from build123d import *

# Parameters (mm, degrees)
SKETCH8_R           = 2.38125
SKETCH8_R_2         = 1.82245
SKETCH10_R          = 2.38125
BOSS_EXTRUDE3_DEPTH = 1.778
BOSS_EXTRUDE3_TAPER = -37
SKETCH11_R          = 1.82245
CUT_EXTRUDE2_DEPTH  = 2.7780001
CUT_EXTRUDE2_TAPER  = -37


with BuildPart() as part:
    # Sweep2: sweep along a path in Sketch9
    with BuildLine(Plane(origin=(0, 0, 0), x_dir=(0, 0, -1), z_dir=(1, 0, 0))) as sweep2_path:
        Line((-19.702223994, -95.902223994), (-19.702223994, -19.702223994))
        ThreePointArc((-19.702223994, -19.702223994), (-13.931576191, -5.770647803), (0, 0))
    # Sketch8 → Sweep2 (sweep)
    with BuildSketch(Plane.XY):
        Circle(SKETCH8_R)
        Circle(SKETCH8_R_2, mode=Mode.SUBTRACT)
    sweep2 = sweep(path=sweep2_path.line)

    # Sketch10 → Boss-Extrude3 (add)
    with BuildSketch(Plane.XZ.offset(95.902223994)):
        with Locations((0, 19.702223994)):
            Circle(SKETCH10_R)
    boss_extrude3 = extrude(amount=BOSS_EXTRUDE3_DEPTH, taper=BOSS_EXTRUDE3_TAPER)

    # Sketch11 → Cut-Extrude2 (cut, through all)
    with BuildSketch(Plane(origin=(0, -95.902223994, 0), x_dir=(1, 0, 0), z_dir=(0, 1, 0))):
        with Locations(Location((0, -19.702223994, 0), (0, 0, 270))):  # turned: the seam where the file's is
            Circle(SKETCH11_R)
    cut_extrude2 = extrude(amount=-CUT_EXTRUDE2_DEPTH, taper=CUT_EXTRUDE2_TAPER, mode=Mode.SUBTRACT)

    # Mirror1: Sweep2, Boss-Extrude3, Cut-Extrude2 across plane
    add(sweep2.mirror(Plane.XY))
    add(boss_extrude3.mirror(Plane.XY))
    add(cut_extrude2.mirror(Plane.XY), mode=Mode.SUBTRACT)


solid = part.part
Source: CAD feature listing. Evaluate the final solid. Frame: model axes, mm. A direction names the side the tool comes from. Round coordinates to 2 decimals unless told otherwise and drop trailing zeros. Loops run counter-clockwise (first coordinate to the right, second up) from the corner with the lowest first, then second, coordinate; pieces in that order, holes last. Notation, with made-up numbers: (-4.5, 45.25) - (23.5, 45.25) arc R36 cw to (23.5, 79.25) - close; hole circle Ø4 at (-29.75, -36). An arc over 180 degrees is marked (long way). Write item = value, one per line. Start each with the question number.
(1) Section query B-B, the plane y = -12.5. State how many separate pieces and enclosed holes the cut face has, plus the area to 3 significant figures.
(2) Ray query, line 1 along Z through (x, y) = (-0.25, -37.5); line 2 along X through (y, z) = (-33, 19.5); line 3 along Z through (x, y) = (-0.5, -71). Return the intervals inside material, ascending. Write a range as from..to.
(3) Pull-direction query (Z, two-part tool) for faces 3 (the face through (-0.237, -57.269, -17.895)), 4 (the face through (-0.237, -57.269, 17.895)), 5 (the face through (-2, -97.68, -17)); classes: +Z half, -Z half, draft (parallel to the pull), parting line (faces both ways), or undercut.
(4) Pin query (flat end, axial travel): pin 1 (3.5 mm diameter, centred on x = 0, z = -19.7, fed in from +Y); pin 2 (1.5 mm diameter, centred on x = -1, y = -37, fed in from -Z); pin 3 (4 mm diameter, centred on x = 0, y = -48.5, fed in from +Z). Return the tip coordinate at first contact, or that it passes through.
(5) Set-up query: faces 1 (the face through (-2, -97.68, 17)), 2 (the face through (1.099, -57.269, -21.815)). Return all of +Z, -Z, +X, -X, +Y, -Y with unobstructed straight access to the full face (end or side cutting, diameter ignored); none if empty.
(6) Section query A-A, the plane y = -41. Output: boundary loops of the cut face in (x, z), plus the area to 3 significant figures.
Conclusion:
q1.separate_pieces = 2
q1.enclosed_holes = 2
q1.area = 15.9 mm2
q2.line_1 = -22.07..-21.51, -17.9..-17.33, 17.33..17.9, 21.51..22.07
q2.line_2 = -2.37..-1.81, 1.81..2.37
q2.line_3 = -22.03..-21.45, -17.95..-17.37, 17.37..17.95, 21.45..22.03
q3.face_3 = undercut
q3.face_4 = undercut
q3.face_5 = draft
q4.pin_1 = -6.84
q4.pin_2 = -22.07
q4.pin_3 = 22.08
q5.face_1 = +Z, -Z, +X, -X, -Y
q5.face_2 = none
q6.outline = circle Ø4.76 at (0, -19.7); circle Ø4.76 at (0, 19.7); hole circle Ø3.64 at (0, -19.7); hole circle Ø3.64 at (0, 19.7)
q6.area = 14.8 mm2
